from build123d import *

# Parameters (mm, degrees)
F0_R     = 17.5
F0_R_2   = 3.6
F1_DEPTH = 13
F4_SIZE2 = 1.25
F4_SIZE  = 3.25


with BuildPart() as f1:
    # F0 (on Top) → F1 (new body)
    with BuildSketch(Plane.XY):
        Circle(F0_R)
        Circle(F0_R_2, mode=Mode.SUBTRACT)
    extrude(amount=F1_DEPTH)

    # F2 (on Front) → F3 (revolve, cut)
    with BuildSketch(Plane.XZ):
        Polygon((17.5, 2), (17.5, 11), (14.5, 6.5113911405), align=None)
    revolve(axis=Axis((0, 0, 0), (0, 0, 1)), mode=Mode.SUBTRACT)

    # F4
    f4_edges = [f1.edges().sort_by_distance(p)[0] for p in [
        (-3.6, 0, 13),
        (-3.6, 0, 0),
    ]]
    f4_side = f1.faces().sort_by_distance((-3.6, 0, 6.5))[0]
    chamfer(f4_edges, length=F4_SIZE, length2=F4_SIZE2, reference=f4_side)


solid = f1.part
Check sheet for the modelled part. Datum: model origin and axes. Units: mm. A direction names the side the tool comes from. Give positions to 0.01 mm unless a question says otherwise; leave off trailing zeros. Write each loop counter-clockwise with the first axis right and the second up, starting at its lowest first coordinate (ties: lowest second). Pieces come first, ordered by that corner, then holes. Notation, with made-up numbers: M 21,-5 L 68,-5 A19 ccw 68,13 Z; hole C 39.25,-7 d3. An arc over 180 degrees is marked long. Use one line per item in the form item = value.
(1) Material ranges on line 1 along Y through (x, z) = (0, 6.25); line 2 along Y through (x, z) = (2.5, 2.5); line 3 along X through (y, z) = (-2.5, 3.75), recorded low to high.
Answer block:
line_1 = -14.67 to -3.6, 3.6 to 14.67
line_2 = -16.98 to -2.98, 2.98 to 16.98
line_3 = -16.14 to -2.59, 2.59 to 16.14
(2) Draft check along Y on faces 3 (the conical face through (3.51, 1.1, 9.95)), 4 (the flat face through (4, -4, 0)), 5 (the conical face through (13.97, 4.4, 6.73)). Enter one of: pulls with the +Y half, pulls with the -Y half, needs draft (parallel to the pull), parting line crosses it, or undercut.
Answer block:
face_3 = undercut
face_4 = needs draft
face_5 = parting line crosses it
(3) Depth check by flat-ended pin: P1, Ø6, axis at y = -8, z = 5.5, coming from the -X side; P2, Ø2, axis at x = 5.5, z = 8, coming from the -Y side; P3, Ø5, axis at x = -4.5, z = 9.5, coming from the +Y side. Enter the tip coordinate at first touch or a pass-through.
Answer block:
P1 = -15.6
P2 = -15.28
P3 = 17.32
(4) Section check C-C on z = 2.5. Record the boundary of the cut face in (x, y), plus the area to 3 significant figures.
Answer block:
outline = C 0,0 d34.34; hole C 0,0 d7.78
area = 878 mm2
(5) Section check D-D on z = 7.25. Record the boundary of the cut face in (x, y).
Answer block:
outline = C 0,0 d29.99; hole C 0,0 d7.2
(6) Tool access check on faces 1 (the cylindrical face through (3.434, 1.081, 6.454)), 2 (the conical face through (-3.18, -14.34, 6.23)). Record the directions out of +Z, -Z, +X, -X, +Y, -Y that give a thin tool (end or side, any length) a straight path to the whole face; none if there is none.
Answer block:
face_1 = +Z, -Z
face_2 = none
(7) Section check A-A on x = 0. Record the boundary of the cut face in (y, z), plus the area to 3 significant figures.
Answer block:
outline = M -17.5,0 L -4.85,0 L -3.6,3.25 L -3.6,9.75 L -4.85,13 L -17.5,13 L -17.5,11 L -14.5,6.51 L -17.5,2 Z; M 3.6,3.25 L 4.85,0 L 17.5,0 L 17.5,2 L 14.5,6.51 L 17.5,11 L 17.5,13 L 4.85,13 L 3.6,9.75 Z
area = 326 mm2
